Work out the finished part from the listing and answer in its coordinate system (mm). Coordinates: 2 decimals unless noted, no trailing zeros. Loops run counter-clockwise (first coordinate to the right, second up) from the corner with the lowest first, then second, coordinate; pieces in that order, holes last. Notation, with made-up numbers: (-23.5, 33.25) -> (11.5, 33.25) arc R25 ccw to (11.5, 61.25) -> close; hole circle Ø10 at (-23.75, 29.25). An arc over 180 degrees is marked (long way). Use a Markdown table: item, result.
Autodesk Inventor part; units mm, degrees
ref_plane "YZ Plane" through (0, 0, 0) normal (1, 0, 0) x (0, 1, 0)
ref_plane "XZ Plane" through (0, 0, 0) normal (0, 1, 0) x (-1, 0, 0)
ref_plane "XY Plane" through (0, 0, 0) normal (0, 0, 1) x (1, 0, 0)
sketch "Sketch1" plane through (0, 0, 0) normal (0, 0, 1) x (1, 0, 0)
  line L0 (0, 0) -> (279.4, 0)
  line L1 (279.4, 0) -> (279.4, 25.4)
  line L2 (279.4, 25.4) -> (0, 25.4)
  line L3 (0, 25.4) -> (0, 0)
  dimension "d2" = 279.4
  dimension "d3" = 25.4
extrude "Extrusion1" add sketch "Sketch1" along normal blind 2.54
sketch "Sketch2" plane through (0, 0, 0) normal (0, 0, -1) x (-1, 0, 0)
  circle A0 centre (-12.7, 12.7) radius 2.5797
  line L0 (0, 25.4) -> (0, 0)
  line L1 (0, 0) -> (-279.4, 0)
  dimension "d6" = 5.1594
  dimension "d7" = 12.7
  dimension "d8" = 12.7
extrude "Extrusion2" cut sketch "Sketch2" against normal blind 25.4
sketch "Sketch3" plane through (0, 0, 2.54) normal (0, 0, 1) x (1, 0, 0)
  circle A0 centre (266.7, 12.7) radius 2.5797
  line L0 (279.4, 0) -> (279.4, 25.4)
  line L1 (0, 0) -> (279.4, 0)
  dimension "d11" = 5.1594
  dimension "d12" = 12.7
  dimension "d13" = 12.7
extrude "Extrusion3" cut sketch "Sketch3" against normal blind 25.4
properties part number "supports"
Q1. Determine the mould class of faces 1 (the cylindrical face through (10.317, 11.712, 1.252)), 2 (the flat face through (138, 13, 0)), 3 (the cylindrical face through (264.123, 12.813, 1.288)) for opening direction Y: pulls with the +Y half, pulls with the -Y half, needs draft (parallel to the pull), parting line crosses it, or undercut.
Solved:
| item | result |
|---|---|
| face 1 | undercut |
| face 2 | needs draft |
| face 3 | undercut |
Q2. Consider line 1 (X direction, y = 12.5, z = 2.3); line 2 (Y direction, x = 12.7, z = 1.05); line 3 (X direction, y = 11.75, z = 2.1). Determine where each line is inside the solid, lowest interval first. Write a range as [from, to].
Solved:
| item | result |
|---|---|
| line 1 | [0, 10.13], [15.27, 264.13], [269.27, 279.4] |
| line 2 | [0, 10.12], [15.28, 25.4] |
| line 3 | [0, 10.3], [15.1, 264.3], [269.1, 279.4] |
Q3. Section B-B on x = 266.7 is taken. Determine the outline of the cut face in (y, z), and give its area (3 significant figures).
Solved:
| item | result |
|---|---|
| outline | (0, 0) -> (10.12, 0) -> (10.12, 2.54) -> (0, 2.54) -> close; (15.28, 0) -> (25.4, 0) -> (25.4, 2.54) -> (15.28, 2.54) -> close |
| area | 51.4 mm² |
Q4. Section A-A on y = 12.7 is taken. Determine the outline of the cut face in (x, z), and give its area (3 significant figures).
Solved:
| item | result |
|---|---|
| outline | (0, 0) -> (10.12, 0) -> (10.12, 2.54) -> (0, 2.54) -> close; (15.28, 0) -> (264.12, 0) -> (264.12, 2.54) -> (15.28, 2.54) -> close; (269.28, 0) -> (279.4, 0) -> (279.4, 2.54) -> (269.28, 2.54) -> close |
| area | 683 mm² |
